Could you check a few things on this model? Use its own coordinates, in mm. Give positions to 0.01 mm unless a question says otherwise; leave off trailing zeros. Loops run counter-clockwise (first coordinate to the right, second up) from the corner with the lowest first, then second, coordinate; pieces in that order, holes last. Notation, with made-up numbers: M -14.5,-34.75 L -2.5,-34.75 A19 cw -2.5,-29.75 Z; hole C -32,-30.75 d9. An arc over 180 degrees is marked long. Use CSV: the item, a comma, the result in double quotes.
```python
from build123d import *

# Parameters (mm, degrees)
F0_R     = 2.5527
F1_DEPTH = 3.175
F2_R     = 3.175


with BuildPart() as f1:
    # F0 (on Top) → F1 (new body)
    with BuildSketch(Plane.XY):
        Polygon((12.7, 63.5), (-12.7, 63.5), (-12.7, -12.7), (63.5, -12.7), (63.5, 12.7), align=None)
        Circle(F0_R, mode=Mode.SUBTRACT)
        with Locations((12.7, 0)):
            Circle(F0_R, mode=Mode.SUBTRACT)
        with Locations((25.4, 0)):
            Circle(F0_R, mode=Mode.SUBTRACT)
        with Locations((0, 12.7)):
            Circle(F0_R, mode=Mode.SUBTRACT)
        with Locations((0, 25.4)):
            Circle(F0_R, mode=Mode.SUBTRACT)
        with Locations((38.1, 0)):
            Circle(F0_R, mode=Mode.SUBTRACT)
        with Locations((50.8, 0)):
            Circle(F0_R, mode=Mode.SUBTRACT)
        with Locations((0, 38.1)):
            Circle(F0_R, mode=Mode.SUBTRACT)
        with Locations((0, 50.8)):
            Circle(F0_R, mode=Mode.SUBTRACT)
    extrude(amount=F1_DEPTH)

    # F2
    f2_edges = [f1.edges().sort_by_distance(p)[0] for p in [
        (-12.7, 63.5, 1.5875),
        (12.7, 63.5, 1.5875),
        (-12.7, -12.7, 1.5875),
        (63.5, -12.7, 1.5875),
        (63.5, 12.7, 1.5875),
    ]]
    fillet(f2_edges, radius=F2_R)


solid = f1.part
```
1. I'm going to push a flat-ended pin straight in: pin 1 Ø6.5 at (x, y) = (0, 50.8) entering from -Z. Where does the tip first touch, or does it pass through?
Outcome:
pin 1,"z = 0"
2. Please list where these lines run through material, in increasing order: line 1 (Y direction, x = 0, z = 1.75); line 2 (Y direction, x = -1, z = 2.15); line 3 (Y direction, x = 36, z = 0.25).
Outcome:
line 1,"-12.7 to -2.55, 2.55 to 10.15, 15.25 to 22.85, 27.95 to 35.55, 40.65 to 48.25, 53.35 to 63.5"
line 2,"-12.7 to -2.35, 2.35 to 10.35, 15.05 to 23.05, 27.75 to 35.75, 40.45 to 48.45, 53.15 to 63.5"
line 3,"-12.7 to -1.45, 1.45 to 40.2"
3. I want a section at A-A, the plane z = 2.45. Give the number of separate pieces and of enclosed holes in the cut face, then the cut area to 3 significant figures.
Outcome:
separate pieces,"1"
enclosed holes,"9"
area,"4,320 mm2"
4. I want a section at B-B, the plane x = 0. List the corners of the cut face in (y, z) for me (3 decimals).
Outcome:
outline,"M -12.7,0 L -2.553,0 L -2.553,3.175 L -12.7,3.175 Z; M 2.553,0 L 10.147,0 L 10.147,3.175 L 2.553,3.175 Z; M 15.253,0 L 22.847,0 L 22.847,3.175 L 15.253,3.175 Z; M 27.953,0 L 35.547,0 L 35.547,3.175 L 27.953,3.175 Z; M 40.653,0 L 48.247,0 L 48.247,3.175 L 40.653,3.175 Z; M 53.353,0 L 63.5,0 L 63.5,3.175 L 53.353,3.175 Z"
5. If we mould it in two halves opening along X, with no side actions, what happens to faces 1 (the face through (63.5, 1, 2)), 2 (the face through (16, 17, 0)), 3 (the face through (48.25, 0.11, 1.57))? For each: +X half, -X half, draft (parallel to the pull), parting line (faces both ways), or undercut.
Outcome:
face 1,"+X half"
face 2,"draft"
face 3,"undercut"
6. I want a section at D-D, the plane x = 38.1. List the corners of the cut face in (y, z) for me (3 decimals).
Outcome:
outline,"M -12.7,0 L -2.553,0 L -2.553,3.175 L -12.7,3.175 Z; M 2.553,0 L 38.1,0 L 38.1,3.175 L 2.553,3.175 Z"
